Verification items for the finished model (mm, model axes). A direction names the side the tool comes from. Coordinates: 2 decimals unless noted, no trailing zeros. Loops run counter-clockwise (first coordinate to the right, second up) from the corner with the lowest first, then second, coordinate; pieces in that order, holes last.
Q1. Mould release check, pull along Y, two halves, no side actions. Record for faces 3 (the face through (10.93, -1.11, 0.2)), 4 (the face through (0, 0, 1.4)), 5 (the face through (10.93, 1.11, 0.2)), 6 (the face through (10.85, -0.04, 0.2)): +Y half, -Y half, draft (parallel to the pull), parting line (faces both ways), or undercut.
Q2. Go/stop test with flat-tipped pins: P1, Ø3, axis at x = 9.85, y = 0, coming from the -Z side; P2, Ø0.7, axis at x = -0.5, y = -4, coming from the +Z side; P3, Ø3, axis at x = 5, y = 2, coming from the +Z side. Record where each tip stops, or that it passes through.
Q3. Access from +Z, -Z, +X, -X, +Y, -Y to the whole of each face (thin tool, end or side, straight path). Record for faces 1 (the face through (3, 0, 0.4)), 2 (the face through (1, 0, 0)).
Q4. Material ranges on probe 1 along X at (y, z) = (0, 0.3); probe 2 along Y at (x, z) = (9.85, 0.2); probe 3 along Z at (x, y) = (4.25, -4.25), recorded low to high.
Q5. Sectioned sample at B-B (x = 8). Enter the section's corners in (y, z), then the cut area to 3 significant figures.
Autodesk Fusion 360 part; units mm, degrees
sketch "Base" plane through (0, 0, 0) normal (0, 0, 1) x (1, 0, 0) in component "Positive Connector"
  line L0 (4.7, -4.95) -> (-4.7, -4.95)
  line L1 (-4.7, -4.95) -> (-4.7, 4.95)
  line L2 (-4.7, 4.95) -> (4.7, 4.95)
  line L3 (4.7, 4.95) -> (4.7, -4.95)
  line L4 (4.7, -4.95) -> (-4.7, 4.95) construction
  line L5 (-4.7, -4.95) -> (4.7, 4.95) construction
  dimension "d1" = 9.4
  dimension "d2" = 9.9
extrude "Extrude1" add sketch "Base" along normal blind 0.4 in component "Positive Connector"
fillet "Fillet1" radius 0.5 4 edges at (4.7, -4.95, 0.2) (4.7, 4.95, 0.2) (-4.7, 4.95, 0.2) (-4.7, -4.95, 0.2) in component "Positive Connector"
sketch "Connector" plane through (4.7, 0, 0) normal (1, 0, 0) x (0, 1, 0) in component "Positive Connector"
  line L0 (4.45, 0) -> (4.45, 0.4)
  line L1 (4.45, 0.4) -> (-4.45, 0.4)
  line L2 (-4.45, 0.4) -> (-4.45, 0)
  line L3 (-4.45, 0) -> (4.45, 0)
  line L4 (-4.45, 0.2) -> (4.45, 0.2) construction
  line L5 (1.55, 0) -> (-1.55, 0)
  line L6 (-1.55, 0) -> (-1.55, 0.4)
  line L7 (-1.55, 0.4) -> (1.55, 0.4)
  line L8 (1.55, 0.4) -> (1.55, 0)
  line L9 (1.55, 0) -> (-1.55, 0.4) construction
  line L10 (-1.55, 0) -> (1.55, 0.4) construction
  point P0 (0, 0.2)
  dimension "d6" = 3.1
extrude "Extrude2" add sketch "Connector" along normal blind 6.7 contours L1 L3 L5 L6 L7 L8 in component "Positive Connector"
fillet "Fillet2" radius 1.55 2 edges at (11.4, -1.55, 0.2) (11.4, 1.55, 0.2) in component "Positive Connector"
sketch "Taps" plane through (0, 0, 0.4) normal (0, 0, 1) x (-1, 0, 0) in component "Positive Connector"
  arc A0 (-9.85, 1.55) -> (-9.85, -1.55) centre (-9.85, 0) ccw
  line L0 (-9.85, -1.55) -> (-4.7, -1.55)
  line L1 (-4.7, -1.55) -> (-4.7, -4.45)
  arc A1 (-4.7, -4.45) -> (-4.2, -4.95) centre (-4.2, -4.45) ccw
  line L2 (-4.2, -4.95) -> (4.2, -4.95)
  arc A2 (4.2, -4.95) -> (4.7, -4.45) centre (4.2, -4.45) ccw
  line L3 (4.7, -4.45) -> (4.7, 4.45)
  arc A3 (4.7, 4.45) -> (4.2, 4.95) centre (4.2, 4.45) ccw
  line L4 (4.2, 4.95) -> (-4.2, 4.95)
  arc A4 (-4.2, 4.95) -> (-4.7, 4.45) centre (-4.2, 4.45) ccw
  line L5 (-4.7, 4.45) -> (-4.7, 1.55)
  line L6 (-4.7, 1.55) -> (-9.85, 1.55)
  line L7 (4.7, 0) -> (-11.4, 0) construction
  line L8 (-9.85, -1.55) -> (-9.85, 1.55) construction
  circle A5 centre (-9.85, 0) radius 1
  line L9 (0, -4.95) -> (0, 4.95) construction
  circle A6 centre (0, 0) radius 2.5
  line L10 (-0.6, -3.05) -> (0.6, -3.05)
  line L11 (0.6, -3.05) -> (0.6, -4.55)
  line L12 (0.6, -4.55) -> (-0.6, -4.55)
  line L13 (-0.6, -4.55) -> (-0.6, -3.05)
  line L14 (-0.6, -3.05) -> (0.6, -4.55) construction
  line L15 (0.6, -3.05) -> (-0.6, -4.55) construction
  line L16 (-0.6, 4.55) -> (0.6, 4.55)
  line L17 (0.6, 4.55) -> (0.6, 3.05)
  line L18 (0.6, 3.05) -> (-0.6, 3.05)
  line L19 (-0.6, 3.05) -> (-0.6, 4.55)
  line L20 (-0.6, 4.55) -> (0.6, 3.05) construction
  line L21 (0.6, 4.55) -> (-0.6, 3.05) construction
  point P0 (0, -3.8)
  point P1 (0, 3.8)
  dimension "d10" = 1.55
  dimension "d11" = 2
  dimension "d12" = 5
  dimension "d13" = 1.2
  dimension "d14" = 1.5
  dimension "d15" = 0.4
  dimension "d16" = 1.2
  dimension "d17" = 1.5
  dimension "d18" = 0.4
extrude "Extrude3" cut sketch "Taps" against normal up to surface (0.4 mm away) contours A5 in component "Positive Connector"
extrude "Extrude4" add sketch "Taps" along normal blind 0.6 contours L10 L11 L12 L13 | L16 L17 L18 L19 in component "Positive Connector"
fillet "Fillet3" radius 0.6 2 edges at (0.6, 3.8, 1) (0.6, -3.8, 1) in component "Positive Connector"
extrude "Extrude5" add sketch "Taps" along normal blind 1 contours A6 in component "Positive Connector"
fillet "Fillet4" radius 1 1 edges at (2.3308, 0.904, 1.4) in component "Positive Connector"
component "Positive Connector" placed x (1, 0, 0) y (0, 1, 0) z (0, 0, 1) at (0, 0, 0)
Geometry check:
1. face 3: -Y half
1. face 4: draft
1. face 5: +Y half
1. face 6: undercut
2. P1: stops at z = 0
2. P2: stops at z = 1
2. P3: stops at z = 0.4
3. face 1: +Z
3. face 2: -Z, +X, -X, +Y, -Y
4. probe 1: x = -4.7 to 8.85, 10.85 to 11.4
4. probe 2: y = -1.55 to -1, 1 to 1.55
4. probe 3: z = 0 to 0.4
5. outline: (-1.55, 0) - (1.55, 0) - (1.55, 0.4) - (-1.55, 0.4) - close
5. area: 1.24 mm2
